```python
from build123d import *

# Parameters (mm, degrees)
F0_W     = 101.6
F0_H     = 25.4
F1_DEPTH = 3.175
F2_SIZE  = 3.17499
F3_SIZE  = 3.17499


# Not quite as in the source:
# - a fillet or chamfer is up to 0.001 mm smaller than in the source, because OpenCascade refuses the exact size
# - a length typed as a fraction of an inch, garbled in the dataset ("3 / 203.2 mm" for 3/8 in), is restored


with BuildPart() as f1:
    # F0 (on Top) → F1 (new body)
    with BuildSketch(Plane.XY):
        Rectangle(F0_W, F0_H)
    extrude(amount=F1_DEPTH)

    # F2 (size 3.175 in the source; OpenCascade refuses exactly that, so slightly less here)
    f2_edges = [f1.edges().sort_by_distance(p)[0] for p in [
        (0, 12.7, 3.175),
    ]]
    chamfer(f2_edges, length=F2_SIZE)

    # F3 (size 3.175 in the source; OpenCascade refuses exactly that, so slightly less here)
    f3_edges = [f1.edges().sort_by_distance(p)[0] for p in [
        (0, -12.7, 0),
    ]]
    chamfer(f3_edges, length=F3_SIZE)


solid = f1.part
```
The listing builds one solid part. Answer for the finished solid, in the listing's coordinates (mm). Round coordinates to 2 decimals unless told otherwise and drop trailing zeros. Loops run counter-clockwise (first coordinate to the right, second up) from the corner with the lowest first, then second, coordinate; pieces in that order, holes last.
Q1. Section B-B, the plane y = 10.75 is taken. Determine the outline of the cut face in (x, z), then the cut area to 3 significant figures.
Q2. Section C-C, the plane z = 2.6 is taken. Determine the outline of the cut face in (x, y) (3 decimals), then the cut area to 3 significant figures.
Q3. Find the intervals of material crossed by line 1 (Z direction, x = 2.5, y = 11); line 2 (Y direction, x = -6, z = 0.7) (3 decimals); line 3 (Y direction, x = 7, z = 2.1) (3 decimals), in increasing order.
Completed:
1. outline: (-50.8, 0) - (50.8, 0) - (50.8, 1.95) - (-50.8, 1.95) - close
1. area: 198 mm2
2. outline: (-50.8, -12.125) - (50.8, -12.125) - (50.8, 10.1) - (-50.8, 10.1) - close
2. area: 2,260 mm2
3. line 1: z = 0 to 1.7
3. line 2: y = -10.225 to 12
3. line 3: y = -11.625 to 10.6
